```python
from build123d import *

# Parameters (mm, degrees)
SKETCH038_R = 1.6
PAD_DEPTH   = 5


with BuildPart() as part:
    # Sketch038 → Pad (new body)
    with BuildSketch(Plane.XY):
        with BuildLine():
            ThreePointArc((4, 0), (0, 4), (-4, 0))
            Line((-4, 0), (-4, -54.5))
            ThreePointArc((-14, -64.5), (-6.928932, -61.571068), (-4, -54.5))
            Line((-14, -64.5), (-20, -64.5))
            ThreePointArc((-20, -64.5), (-23.535534, -65.964466), (-25, -69.5))
            Line((-25, -69.5), (-25, -103.46))
            ThreePointArc((-28.54, -107), (-26.036842, -105.963158), (-25, -103.46))
            Line((-98.92301, -107), (-28.54, -107))
            ThreePointArc((-98.92301, -107), (-101.113722, -107.201662), (-103.230804, -107.79987))
            ThreePointArc((-107.79987, -103.230804), (-107, -107), (-103.230804, -107.79987))
            ThreePointArc((-107.79987, -103.230804), (-107.201662, -101.113722), (-107, -98.92301))
            Line((-107, 98.92301), (-107, -98.92301))
            ThreePointArc((-107, 98.92301), (-107.201662, 101.113722), (-107.79987, 103.230804))
            ThreePointArc((-103.230804, 107.79987), (-107, 107), (-107.79987, 103.230804))
            ThreePointArc((-103.230804, 107.79987), (-101.113722, 107.201662), (-98.92301, 107))
            Line((98.92301, 107), (-98.92301, 107))
            ThreePointArc((98.92301, 107), (101.113722, 107.201662), (103.230804, 107.79987))
            ThreePointArc((107.79987, 103.230804), (107, 107), (103.230804, 107.79987))
            ThreePointArc((107.79987, 103.230804), (107.201662, 101.113722), (107, 98.92301))
            Line((107, -98.92301), (107, 98.92301))
            ThreePointArc((107, -98.92301), (107.201662, -101.113722), (107.79987, -103.230804))
            ThreePointArc((103.230804, -107.79987), (107, -107), (107.79987, -103.230804))
            ThreePointArc((103.230804, -107.79987), (101.113722, -107.201662), (98.92301, -107))
            Line((28.54, -107), (98.92301, -107))
            ThreePointArc((25, -103.46), (26.036842, -105.963158), (28.54, -107))
            Line((25, -103.46), (25, -69.5))
            ThreePointArc((25, -69.5), (23.535534, -65.964466), (20, -64.5))
            Line((20, -64.5), (14, -64.5))
            ThreePointArc((4, -54.5), (6.928932, -61.571068), (14, -64.5))
            Line((4, -54.5), (4, 0))
        make_face()
        with Locations((104.5, -104.5)):
            Circle(SKETCH038_R, mode=Mode.SUBTRACT)
        with Locations((104.5, 104.5)):
            Circle(SKETCH038_R, mode=Mode.SUBTRACT)
        with Locations((-104.5, -104.5)):
            Circle(SKETCH038_R, mode=Mode.SUBTRACT)
        with Locations((71, -65)):
            Circle(SKETCH038_R, mode=Mode.SUBTRACT)
        with Locations((71, 65)):
            Circle(SKETCH038_R, mode=Mode.SUBTRACT)
        with Locations((-104.5, 104.5)):
            Circle(SKETCH038_R, mode=Mode.SUBTRACT)
        with Locations((-71, -65)):
            Circle(SKETCH038_R, mode=Mode.SUBTRACT)
        with Locations((-71, 65)):
            Circle(SKETCH038_R, mode=Mode.SUBTRACT)
    extrude(amount=PAD_DEPTH)


solid = part.part
```
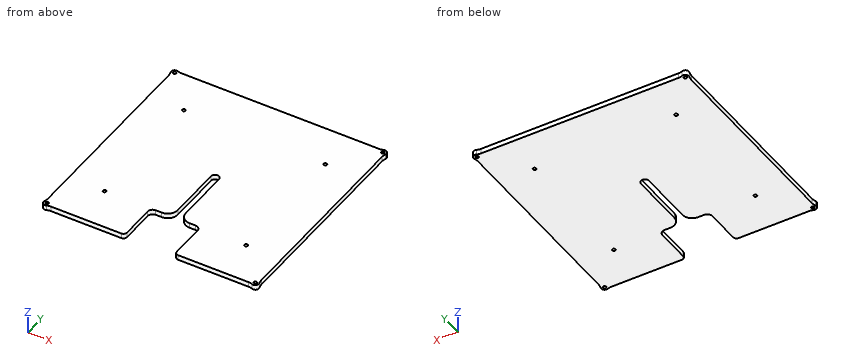
Build history of the part. All positions in model axes, mm. Round coordinates to 2 decimals unless told otherwise and drop trailing zeros. Write each loop counter-clockwise with the first axis right and the second up, starting at its lowest first coordinate (ties: lowest second). Pieces come first, ordered by that corner, then holes.
1) Band-saw the part on B-B, the plane x = 0. List the corners of the cut face in (y, z).
2) Pin check, flat tips, straight feed: pin 1 (10 mm diameter, centred on x = 61.5, y = 30.5, fed in from -Z); pin 2 (1.5 mm diameter, centred on y = -6, z = 3.5, fed in from +X); pin 3 (1.5 mm diameter, centred on x = -17, z = 3.5, fed in from -Y); pin 4 (1.5 mm diameter, centred on x = 52, z = 2.5, fed in from -Y). Stop position of each tip, or through.
3) Drill centre lines: probe 1 along Y at (x, z) = (71, 2.45); probe 2 along X at (y, z) = (65, 3.45); probe 3 along Y at (x, z) = (-104.5, 2.75). Where is each one in solid material? Low to high.
4) Band-saw the part on D-D, the plane y = -36. List the corners of the cut face in (x, z).
5) Band-saw the part on A-A, the plane y = -82. List the corners of the cut face in (x, z).
6) Band-saw the part on C-C, the plane z = 2.7. Give the number of separate pieces and of enclosed holes in the cut face, and give its area (3 significant figures).
Ans:
1. outline: (4, 0) - (107, 0) - (107, 5) - (4, 5) - close
2. pin 1: stops at z = 0
2. pin 2: stops at x = 107
2. pin 3: stops at y = -64.5
2. pin 4: stops at y = -107
3. probe 1: y = -107 to -66.6, -63.4 to 63.4, 66.6 to 107
3. probe 2: x = -107 to -72.6, -69.4 to 69.4, 72.6 to 107
3. probe 3: y = -108.04 to -106.1, -102.9 to 102.9, 106.1 to 108.04
4. outline: (-107, 0) - (-4, 0) - (-4, 5) - (-107, 5) - close; (4, 0) - (107, 0) - (107, 5) - (4, 5) - close
5. outline: (-107, 0) - (-25, 0) - (-25, 5) - (-107, 5) - close; (25, 0) - (107, 0) - (107, 5) - (25, 5) - close
6. separate pieces: 1
6. enclosed holes: 8
6. area: 43,100 mm2
